from build123d import *

# Parameters (mm, degrees)
F0_W      = 95.9210544825
F0_H      = 123.1578961015
F1_DEPTH  = 5.8
F2_W      = 14.211
F2_H      = 7.14
F2_W_2    = 14.82887734
F2_H_2    = 7.4144396418
F3_DEPTH  = 18.5
F5_R      = 38.0021383108
F6_DEPTH  = 14
F8_DEPTH  = 13.2
F9_W      = 2.9605254531
F9_H      = 32.5657902285
F10_DEPTH = 40
F12_W     = 106.5789507702
F12_H     = 42.6315842196
F13_DEPTH = 5
F15_W     = 95.0329005718
F15_H     = 31.9736870006
F16_DEPTH = 5
F17_R     = 4.99999
F18_W     = 4.7368425876
F18_H     = 34.638158977
F19_DEPTH = 69.8
F20_W     = 4.737
F20_H     = 34.638
F21_DEPTH = 93.3
F22_W     = 4.737
F22_H     = 34.638
F23_DEPTH = 98.3


# Not quite as in the source:
# - a fillet or chamfer is up to 0.001 mm smaller than in the source, because OpenCascade refuses the exact size


with BuildPart() as f1:
    # F0 (on Top) → F1 (new body)
    with BuildSketch(Plane.XY):
        Rectangle(F0_W, F0_H)
    extrude(amount=F1_DEPTH)

    # F2 (on face) → F3 (join)
    with BuildSketch(Plane.XY.offset(5.8)):
        with Locations((-33.1652933639, 33.6907944659)):
            Rectangle(F2_W, F2_H)
        with Locations((23.060855536, 35.2354664353)):
            Rectangle(F2_W, F2_H)
        with Locations((23.3697903186, -12.0315703675)):
            Rectangle(F2_W, F2_H)
        with Locations((-32.8563585813, -12.2032872729)):
            Rectangle(F2_W_2, F2_H_2)
    extrude(amount=F3_DEPTH)

    # F5 (on offset) → F6 (join)
    with BuildSketch(Plane.XY.offset(19.9)):
        with Locations((-3.2565793954, 6.5131578594)):
            Circle(F5_R)
    extrude(amount=F6_DEPTH)

    # F7 (on face) → F8 (join)
    with BuildSketch(Plane.XY.offset(33.9)):
        with BuildLine():
            Line((30.7933383724, -10.3618418798), (-37.3064971632, -10.3618418798))
            ThreePointArc((-37.3064971632, -10.3618418798), (-36.1766552365, -12.4718657857), (-34.9162250459, -14.5065793768))
            Line((-34.9162250459, -14.5065793768), (28.4030662551, -14.5065793768))
            ThreePointArc((28.4030662551, -14.5065793768), (29.6634964457, -12.4718657857), (30.7933383724, -10.3618418798))
        make_face()
        with BuildLine():
            Line((39.3750034273, -10.3618418798), (30.7933383724, -10.3618418798))
            ThreePointArc((30.7933383724, -10.3618418798), (29.6634964457, -12.4718657857), (28.4030662551, -14.5065793768))
            Line((28.4030662551, -14.5065793768), (39.3750034273, -14.5065793768))
            Line((39.3750034273, -14.5065793768), (39.3750034273, -10.3618418798))
        make_face()
        with BuildLine():
            ThreePointArc((-34.9162250459, -14.5065793768), (-36.1766552365, -12.4718657857), (-37.3064971632, -10.3618418798))
            Line((-37.3064971632, -10.3618418798), (-48.2565825805, -10.3618418798))
            Line((-48.2565825805, -10.3618418798), (-48.2565825805, -14.5065793768))
            Line((-48.2565825805, -14.5065793768), (-34.9162250459, -14.5065793768))
        make_face()
        with BuildLine():
            Line((-37.8681614166, 22.2039483488), (31.3550026259, 22.2039483488))
            ThreePointArc((31.3550026259, 22.2039483488), (30.1557002498, 24.6179109675), (28.7883016181, 26.9407890737))
            Line((28.7883016181, 26.9407890737), (-35.3014604088, 26.9407890737))
            ThreePointArc((-35.3014604088, 26.9407890737), (-36.6688590406, 24.6179109675), (-37.8681614166, 22.2039483488))
        make_face()
        with BuildLine():
            Line((-48.2565825805, 22.2039483488), (-37.8681614166, 22.2039483488))
            ThreePointArc((-37.8681614166, 22.2039483488), (-36.6688590406, 24.6179109675), (-35.3014604088, 26.9407890737))
            Line((-35.3014604088, 26.9407890737), (-48.2565825805, 26.9407890737))
            Line((-48.2565825805, 26.9407890737), (-48.2565825805, 22.2039483488))
        make_face()
        with BuildLine():
            Line((31.3550026259, 22.2039483488), (39.3750034273, 22.2039483488))
            Line((39.3750034273, 22.2039483488), (39.3750034273, 26.9407890737))
            Line((39.3750034273, 26.9407890737), (28.7883016181, 26.9407890737))
            ThreePointArc((28.7883016181, 26.9407890737), (30.1557002498, 24.6179109675), (31.3550026259, 22.2039483488))
        make_face()
    extrude(amount=F8_DEPTH)

    # F9 (on face) → F10 (join)
    with BuildSketch(Plane.XY.offset(33.9)):
        with Locations((-33.7500013411, 5.9210532345)):
            Rectangle(F9_W, F9_H)
        with Locations((26.6447365284, 5.9210532345)):
            Rectangle(F9_W, F9_H)
    extrude(amount=F10_DEPTH)

    # F12 (on offset) → F13 (join)
    with BuildSketch(Plane.XY.offset(73.9)):
        with Locations((-3.5526319407, 7.401315961)):
            Rectangle(F12_W, F12_H)
    extrude(amount=F13_DEPTH)

    # F15 (on face) → F16 (join)
    with BuildSketch(Plane.XY.offset(78.9)):
        with Locations((-3.700658679, 7.105264347)):
            Rectangle(F15_W, F15_H)
    extrude(amount=F16_DEPTH)

    # F17 (radius 5 in the source; OpenCascade refuses exactly that, so slightly less here)
    f17_edges = [f1.edges().sort_by_distance(p)[0] for p in [
        (-3.700659, 23.092108, 83.9),
        (-51.217109, 7.105264, 83.9),
        (-3.700659, -8.881579, 83.9),
        (43.815792, 7.105264, 83.9),
    ]]
    fillet(f17_edges, radius=F17_R)

    # F18 (on face) → F19 (cut)
    with BuildSketch(Plane(origin=(-35.2302640676, 0, 0), x_dir=(0, -1, 0), z_dir=(-1, 0, 0))):
        with Locations((-16.5789490566, 53.742762655)):
            Rectangle(F18_W, F18_H)
    extrude(amount=-F19_DEPTH, mode=Mode.SUBTRACT)

    # F20 (on face) → F21 (cut)
    with BuildSketch(Plane(origin=(-35.2302640676, 0, 0), x_dir=(0, -1, 0), z_dir=(-1, 0, 0))):
        with Locations((-5.8019411517, 54.2707815458)):
            Rectangle(F20_W, F20_H)
    extrude(amount=-F21_DEPTH, mode=Mode.SUBTRACT)

    # F22 (on face) → F23 (cut)
    with BuildSketch(Plane(origin=(-35.2302640676, 0, 0), x_dir=(0, -1, 0), z_dir=(-1, 0, 0))):
        with Locations((5.355990259, 53.9595156418)):
            Rectangle(F22_W, F22_H)
    extrude(amount=-F23_DEPTH, mode=Mode.SUBTRACT)


solid = f1.part
Geometry: final body of the model. Coordinates: model frame, mm. A direction names the side the tool comes from. Coordinates: 2 decimals unless noted, no trailing zeros. Write each loop counter-clockwise with the first axis right and the second up, starting at its lowest first coordinate (ties: lowest second). Pieces come first, ordered by that corner, then holes. Notation, with made-up numbers: (45, 69.25) - (93, 69.25) arc R19 cw to (93, 96.25) - close; hole circle Ø2 at (-23, -11.5). An arc over 180 degrees is marked (long way). Return JSON: item names as keys, results as strings.
Item 1: Reachability of faces 5 (the face through (28.125, 2, 54)), 6 (the face through (35, 25, 33.9)), 7 (the face through (-42, -10.362, 40)), 8 (the face through (-3, -10.362, 40)), 9 (the face through (-34, 8.17, 54)) from +Z, -Z, +X, -X, +Y, -Y: full face, straight path, thin tool, end or side. Return the list, or none.
Completed:
{"face 5": "+X", "face 6": "+X, +Y", "face 7": "-X", "face 8": "none", "face 9": "+X, -X"}
Item 2: Pull-direction query (Z, two-part tool) for faces 1 (the face through (39.375, 25, 40)), 2 (the face through (-7.7, 23.3, 78.9)), 3 (the face through (27, 17, 71.062)), 4 (the face through (-33, 37.261, 15)); classes: +Z half, -Z half, draft (parallel to the pull), parting line (faces both ways), or undercut.
Completed:
{"face 1": "undercut", "face 2": "+Z half", "face 3": "undercut", "face 4": "draft"}
Item 3: Section query D-D (y = -25). Output: boundary loops of the cut face in (x, z).
Completed:
{"outline": "(-47.96, 0) - (47.96, 0) - (47.96, 5.8) - (-47.96, 5.8) - close; (-24.5, 19.9) - (17.98, 19.9) - (17.98, 33.9) - (-24.5, 33.9) - close"}
Item 4: Pin query (flat end, axial travel): pin 1 Ø4.5 at (x, y) = (-16, -11.5) entering from +Z; pin 2 Ø12 at (x, z) = (-36, 68) entering from +Y; pin 3 Ø1.2 at (y, z) = (-11.5, 42.5) entering from +X (3 decimals). Return the tip coordinate at first contact, or that it passes through.
Completed:
{"pin 1": "stops at z = 78.9", "pin 2": "stops at y = 28.72", "pin 3": "stops at x = 39.375"}
Item 5: Line query: L1, parallel to Z at x = -17.5, y = -9; L2, parallel to Z at x = -0.5, y = 16; L3, parallel to Y at x = -35.5, z = 45. Output: solid intervals per line, ascending.
Completed:
{"L1": "z = 0 to 5.8, 19.9 to 33.9, 73.9 to 78.9", "L2": "z = 0 to 5.8, 19.9 to 33.9, 73.9 to 83.9", "L3": "y = -14.51 to -10.36, 22.2 to 26.94"}
Item 6: Section query A-A (z = 56). Count the separate pieces of the cut face and the enclosed holes in it, and give its area (3 significant figures).
Completed:
{"separate pieces": "8", "enclosed holes": "0", "area": "109 mm2"}
